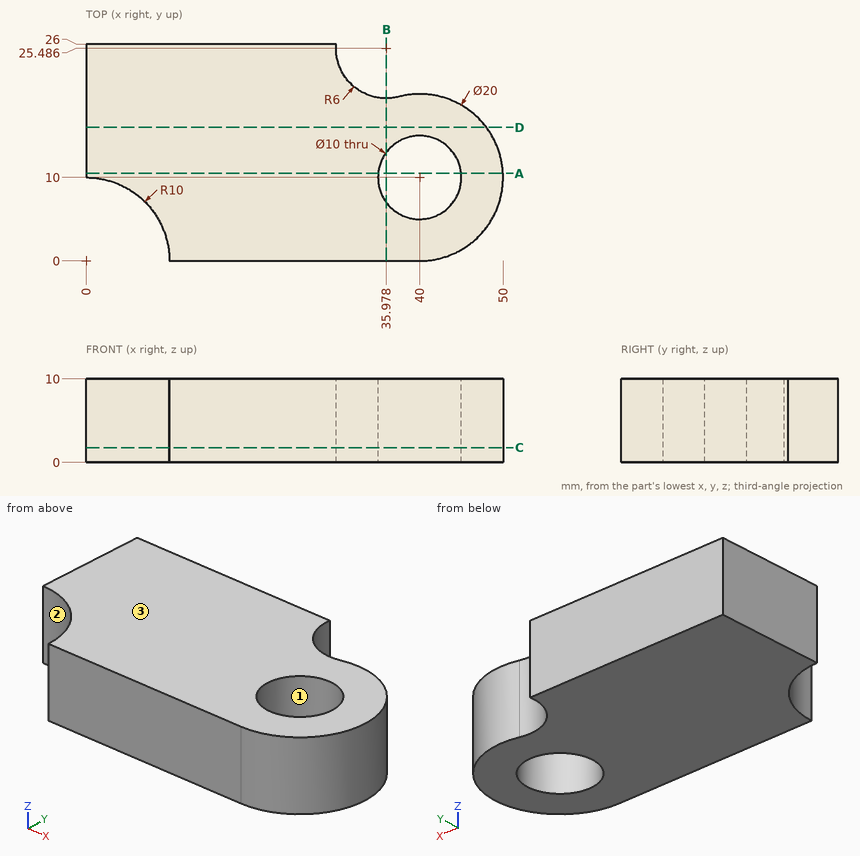
Study the drawing (mm; zero at the part's minimum x, y, z) and answer. Coordinates: 2 decimals unless noted, no trailing zeros. Write each loop counter-clockwise with the first axis right and the second up, starting at its lowest first coordinate (ties: lowest second). Pieces come first, ordered by that corner, then holes. Notation, with made-up numbers: (78.5, 31.25) - (107.5, 31.25) arc R8 cw to (107.5, 35.25) - close; hole circle Ø7 at (66, 58.25). An arc over 180 degrees is marked (long way). Put each result on its own line as item: value.
1. The part is cut by section A-A on y = 10.5. Give the vertices of the cut face in (x, z) (1 decimal), plus the area to 3 significant figures.
Answer sheet:
outline: (0, 0) - (35, 0) - (35, 10) - (0, 10) - close; (45, 0) - (50, 0) - (50, 10) - (45, 10) - close
area: 400 mm^2
2. Find the intervals of material crossed by line 1 along Y through (x, z) = (40, 2.5); line 2 along X through (y, z) = (11.75, 3) (1 decimal); line 3 along Y through (x, z) = (39, 8), in increasing order. Write a range as from..to.
Answer sheet:
line 1: y = 0..5, 15..20
line 2: x = 0..35.3, 44.7..49.8
line 3: y = 0..5.1, 14.9..19.95
3. Determine the mould class of the marked faces 1, 2 and 3 for opening direction Y: pulls with the +Y half, pulls with the -Y half, needs draft (parallel to the pull), parting line crosses it, or undercut.
Answer sheet:
face 1: undercut
face 2: pulls with the -Y half
face 3: needs draft
4. The part is cut by section D-D on y = 16. Give the vertices of the cut face in (x, z), plus the area to 3 significant figures.
Answer sheet:
outline: (0, 0) - (48, 0) - (48, 10) - (0, 10) - close
area: 480 mm^2
5. The part is cut by section C-C on z = 1.75. Give the vertices of the cut face in (x, y).
Answer sheet:
outline: (0, 10) arc R10 cw to (10, 0) - (40, 0) arc R10 ccw (long way) to (37.49, 19.68) arc R6 cw to (30, 26) - (0, 26) - close; hole circle Ø10 at (40, 10)
6. The part is cut by section B-B on x = 36. Give the vertices of the cut face in (y, z), plus the area to 3 significant figures.
Answer sheet:
outline: (0, 0) - (7, 0) - (7, 10) - (0, 10) - close; (13, 0) - (19.49, 0) - (19.49, 10) - (13, 10) - close
area: 135 mm^2
